```python
from build123d import *
from build123d.topology import SkipClean

# Parameters (mm, degrees)
SKETCH_3_R          = 10
CUT_EXTRUDE_1_DEPTH = 2.5


with BuildPart() as part:
    # Sketch 2 → Revolve 7 (revolve)
    with SkipClean():  # the faces are left unmerged after this step: merging them gives an invalid solid
        with BuildSketch(Plane.XY, mode=Mode.PRIVATE) as revolve_7_sk:
            Polygon((5, 11), (0, 11), (0, 0), (5, 0), (5, 3), align=None)
            with BuildLine():
                Line((8, 3), (5, 3))
                Line((5, 3), (5, 0))
                ThreePointArc((5, 0), (7.121320344, 0.878679656), (8, 3))
            make_face()
            Polygon((8, 11), (5, 11), (5, 3), (8, 3), (8, 6.2), align=None)
            with BuildLine():
                Line((11.2, 6.2), (8, 6.2))
                Line((8, 6.2), (8, 3))
                ThreePointArc((8, 3), (10.2627417, 3.9372583), (11.2, 6.2))
            make_face()
            Polygon((33, 11), (8, 11), (8, 6.2), (11.2, 6.2), (29.8, 6.2), (33, 6.2), align=None)
            with BuildLine():
                Line((33, 3), (33, 6.2))
                Line((33, 6.2), (29.8, 6.2))
                ThreePointArc((29.8, 6.2), (30.7372583, 3.9372583), (33, 3))
            make_face()
            Polygon((36, 11), (33, 11), (33, 6.2), (33, 3), (36, 3), (36, 9), align=None)
            with BuildLine():
                Line((37.019323658, 11), (36, 11))
                Line((36, 11), (36, 9))
                Line((36, 9), (37.270805384, 9))
                ThreePointArc((37.270805384, 9), (37.082440651, 9.992125621), (37.019323658, 11))
            make_face()
            with BuildLine():
                ThreePointArc((37.270805384, 13), (37.082440651, 12.007874379), (37.019323658, 11))
                Line((37.019323658, 11), (53.176533665, 11))
                ThreePointArc((53.176533665, 11), (46.105803041, 19.01548801), (37.270805384, 13))
            make_face()
            with BuildLine():
                Line((53.176533665, 11), (37.019323658, 11))
                ThreePointArc((37.019323658, 11), (37.082440651, 9.992125621), (37.270805384, 9))
                ThreePointArc((37.270805384, 9), (46.105803041, 2.98451199), (53.176533665, 11))
            make_face()
        revolve(revolve_7_sk.sketch.rotate(Axis((0, 11, 0), (1, 0, 0)), 270), axis=Axis((0, 11, 0), (1, 0, 0)))
    add(part.part.scale(1), mode=Mode.REPLACE)  # the faces are merged on a copy

    # Sketch 3 → Cut-Extrude 1 (cut)
    with BuildSketch(Plane.ZY):
        with Locations((0, 11)):
            Circle(SKETCH_3_R)
    extrude(amount=-CUT_EXTRUDE_1_DEPTH, mode=Mode.SUBTRACT)


solid = part.part
```
The model under review builds one solid part; all positions refer to its coordinate system, in mm. A direction names the side the tool comes from. Round coordinates to 2 decimals unless told otherwise and drop trailing zeros. Order: outer loops, then holes, each group sorted by start corner. A loop starts at its lowest first (then second) coordinate and runs counter-clockwise, first axis right, second up. Notation, with made-up numbers: M 83.25,16 L 125.25,16 A31 ccw 125.25,54 Z; hole C 89.25,50 d4. An arc over 180 degrees is marked long. Use a Markdown table: item, result.
1) Consider section A-A (y = 11). Write out the cut boundary in (x, z), then the cut area to 3 significant figures.
Report:
| item | result |
|---|---|
| outline | M 0,-11 L 5,-11 A3 ccw 8,-8 A3.2 ccw 11.2,-4.8 L 29.8,-4.8 A3.2 ccw 33,-8 L 36,-8 L 36,-2 L 37.27,-2 A8.08 ccw long 37.27,2 L 36,2 L 36,8 L 33,8 A3.2 ccw 29.8,4.8 L 11.2,4.8 A3.2 ccw 8,8 A3 ccw 5,11 L 0,11 L 0,10 L 2.5,10 L 2.5,-10 L 0,-10 Z |
| area | 652 mm^2 |
2) Consider section B-B (z = 0). Write out the cut boundary in (x, y).
Report:
| item | result |
|---|---|
| outline | M 0,0 L 5,0 A3 ccw 8,3 A3.2 ccw 11.2,6.2 L 29.8,6.2 A3.2 ccw 33,3 L 36,3 L 36,9 L 37.27,9 A8.08 ccw long 37.27,13 L 36,13 L 36,19 L 33,19 A3.2 ccw 29.8,15.8 L 11.2,15.8 A3.2 ccw 8,19 A3 ccw 5,22 L 0,22 L 0,21 L 2.5,21 L 2.5,1 L 0,1 Z |
3) Consider section C-C (x = 13.5). Write out the cut boundary in (y, z), then the cut area to 3 significant figures.
Report:
| item | result |
|---|---|
| outline | C 11,0 d9.6 |
| area | 72.4 mm^2 |
4) Insertion check: pin 1 (1.5 mm diameter, centred on x = 11.5, y = 14, fed in from +Z); pin 2 (1 mm diameter, centred on x = 8, z = 2, fed in from -Y); pin 3 (2 mm diameter, centred on x = 26.5, y = 10.5, fed in from -Z). Each pin has a flat end and moves straight along its axis. Give the tip position at first contact, or say it passes through.
Report:
| item | result |
|---|---|
| pin 1 | z = 5.74 |
| pin 2 | y = 1.54 |
| pin 3 | z = -4.8 |
5) Consider section D-D (y = 4.75). Give the number of separate pieces and of enclosed holes in the cut face, then the cut area to 3 significant figures.
Report:
| item | result |
|---|---|
| separate pieces | 3 |
| enclosed holes | 0 |
| area | 259 mm^2 |
6) Tool access review of faces 1 (the face through (2.5, 11, 0)), 2 (the face through (0, 21, -2)), 3 (the face through (37, 9, 0)): name each direction out of +Z, -Z, +X, -X, +Y, -Y from which nothing blocks a thin tool from reaching the whole face with its end or side.
Report:
| item | result |
|---|---|
| face 1 | -X |
| face 2 | +Z, -Z, -X, +Y, -Y |
| face 3 | none |
7) Draft analysis for pull direction Z (two halves, no side actions). For faces 4 (the face through (36, 13, 2)), 5 (the face through (1.23, 1.24, -2.17)), 6 (the face through (34.52, 18.81, -1.73)), state which applies: released by +Z, released by -Z, zero draft, split by the parting line, or undercut.
Report:
| item | result |
|---|---|
| face 4 | zero draft |
| face 5 | undercut |
| face 6 | split by the parting line |
8) Wall thickness on line 1 along X through (y, z) = (18.25, 0); line 2 along Y through (x, z) = (0.7, 0); line 3 along X through (y, z) = (15.5, -5.5): over which ranges is each line inside the solid? List them lowest first. Write a range as [from, to].
Report:
| item | result |
|---|---|
| line 1 | [2.5, 10.06], [30.94, 36], [41.53, 48.66] |
| line 2 | [0, 1], [21, 22] |
| line 3 | [2.5, 10.22], [30.78, 36], [41.26, 48.94] |
